The model under review builds one solid part; all positions refer to its coordinate system, in mm. Face numbers are marked on the shaded views. A direction names the side the tool comes from. Give positions to 0.01 mm unless a question says otherwise; leave off trailing zeros. Order: outer loops, then holes, each group sorted by start corner. A loop starts at its lowest first (then second) coordinate and runs counter-clockwise, first axis right, second up. Notation, with made-up numbers: M 64,17.25 L 76,17.25 A13 ccw 76,37.25 Z; hole C 23,18.5 d3. An arc over 180 degrees is marked long. One line per question, with ' | ' between items. Start each with the question number.
1. We need section C-C on x = 13. Write out the cut boundary in (y, z).
2. We need section A-A on z = -3. Write out the cut boundary in (x, y), then the cut area to 3 significant figures.
3. Wall thickness on L1, parallel to Z at x = 1, y = 18.5; L2, parallel to X at y = 13.5, z = -5; L3, parallel to Z at x = 10, y = 6 (3 decimals): over which ranges is each line inside the solid? List them lowest first.
4. For the marked faces 1 and 2, list the 3-axis set-ups (+Z, -Z, +X, -X, +Y, -Y) from which the entire face can be reached by the end or side of a thin tool; tool diameter is ignored.
5. The part is to be moulded in two halves that separate along Z. For the marked faces 3, 4 and 5, say which applies: +Z half, -Z half, draft (parallel to the pull), parting line (faces both ways), or undercut.
6. Insertion check: P1, Ø3, axis at x = -2.5, y = 14, coming from the -Z side; P2, Ø12, axis at x = -7.5, y = 7.5, coming from the +Z side; P3, Ø2, axis at y = 5.5, z = -11, coming from the +X side; P4, Ø9, axis at x = 5.56, z = -9.43, coming from the -Y side. Each pin has a flat end and moves straight along its axis. Give the tip position at first contact, or say it passes through.
```python
from build123d import *

# Parameters (mm, degrees)
SKETCH5_R               = 30
BOSS_EXTRUDE1_DEPTH     = 20
SKETCH6_R               = 5.75
CUT_EXTRUDE1_DEPTH      = 50
CUT_EXTRUDE_THIN1_DEPTH = 50
SKETCH11_R              = 1.5
CUT_EXTRUDE2_DEPTH      = 35.227641189


with BuildPart() as part:
    # Sketch5 → Boss-Extrude1 (new body)
    with BuildSketch(Plane(origin=(0, 0, 0), x_dir=(1, 0, 0), z_dir=(0, 1, 0))):
        with Locations(Location((0, 0, 0), (0, 0, 270))):
            Circle(SKETCH5_R)
    extrude(amount=BOSS_EXTRUDE1_DEPTH)

    # Sketch6 → Cut-Extrude1 (cut)
    with BuildSketch(Plane(origin=(0, 20, 0), x_dir=(1, 0, 0), z_dir=(0, 1, 0))):
        with Locations(Location((5.564652455, 9.430649132, 0), (0, 0, 270))):
            Circle(SKETCH6_R)
        with Locations(Location((5.325305202, -9.567843252, 0), (0, 0, 270))):
            Circle(SKETCH6_R)
        with Locations(Location((-11.00819821, 0.138683741, 0), (0, 0, 270))):
            Circle(SKETCH6_R)
    extrude(amount=-CUT_EXTRUDE1_DEPTH, mode=Mode.SUBTRACT)

    # Sketch9 → Cut-Extrude-Thin1 (cut)
    with BuildSketch(Plane(origin=(0, 20, 0), x_dir=(1, 0, 0), z_dir=(0, 1, 0))):
        with BuildLine():
            ThreePointArc((-3.76991423, 9.548248089), (5.682251411, 18.765215817), (14.899219139, 9.313050176))
            Line((14.899219139, 9.313050176), (14.659871887, -9.685442209))
            ThreePointArc((14.659871887, -9.685442209), (5.207706246, -18.902409937), (-4.009261482, -9.450244295))
            Line((-4.009261482, -9.450244295), (-14.008468, -9.324272058))
            ThreePointArc((-14.008468, -9.324272058), (5.081734008, -28.901616455), (24.659078405, -9.811414447))
            Line((24.659078405, -9.811414447), (24.898425657, 9.187077938))
            ThreePointArc((24.898425657, 9.187077938), (5.808223649, 28.764422335), (-13.769120748, 9.674220327))
            Line((-13.769120748, 9.674220327), (-3.76991423, 9.548248089))
        make_face()
        with BuildLine():
            ThreePointArc((10.124185438, -1.49260411), (13.400544345, -14.366723488), (0.526424967, -17.643082394))
            Line((0.526424967, -17.643082394), (-15.807078446, -7.936555401))
            ThreePointArc((-15.807078446, -7.936555401), (-19.083437352, 4.937563977), (-6.209317974, 8.213922883))
            Line((-6.209317974, 8.213922883), (-1.100619557, 16.810503626))
            ThreePointArc((-1.100619557, 16.810503626), (-27.680018096, 10.046262394), (-20.915776863, -16.533136145))
            Line((-20.915776863, -16.533136145), (-4.582273451, -26.239663138))
            ThreePointArc((-4.582273451, -26.239663138), (21.997125088, -19.475421905), (15.232883856, 7.103976633))
            Line((15.232883856, 7.103976633), (10.124185438, -1.49260411))
        make_face()
        with BuildLine():
            ThreePointArc((-6.438623457, -8.011462842), (-19.158344793, -4.430891012), (-15.577772963, 8.288830324))
            Line((-15.577772963, 8.288830324), (0.995077701, 17.580795716))
            ThreePointArc((0.995077701, 17.580795716), (13.714799038, 14.000223886), (10.134227208, 1.280502549))
            Line((10.134227208, 1.280502549), (15.024735309, -7.442050432))
            ThreePointArc((15.024735309, -7.442050432), (22.437352019, 18.890731987), (-3.8954304, 26.303348697))
            Line((-3.8954304, 26.303348697), (-20.468281064, 17.011383305))
            ThreePointArc((-20.468281064, 17.011383305), (-27.880897775, -9.321399113), (-1.548115356, -16.734015824))
            Line((-1.548115356, -16.734015824), (-6.438623457, -8.011462842))
        make_face()
    extrude(amount=-CUT_EXTRUDE_THIN1_DEPTH, mode=Mode.SUBTRACT)


with BuildPart() as cut_extrude_thin1_kept_piece:
    # of the separate pieces the step leaves, the one the design keeps (cut_extrude_thin1_pieces_kept)
    add(part.part.solids().sort_by_distance((-4.009261482, 0, 9.450244295))[0])

    # Sketch11 → Cut-Extrude2 (cut, through all)
    with BuildSketch(Plane(origin=(0, 20, 0), x_dir=(1, 0, 0), z_dir=(0, 1, 0))):
        with Locations(Location((0, 0, 0), (0, 0, 270))):
            Circle(SKETCH11_R)
    extrude(amount=-CUT_EXTRUDE2_DEPTH, mode=Mode.SUBTRACT)


solid = cut_extrude_thin1_kept_piece.part
```
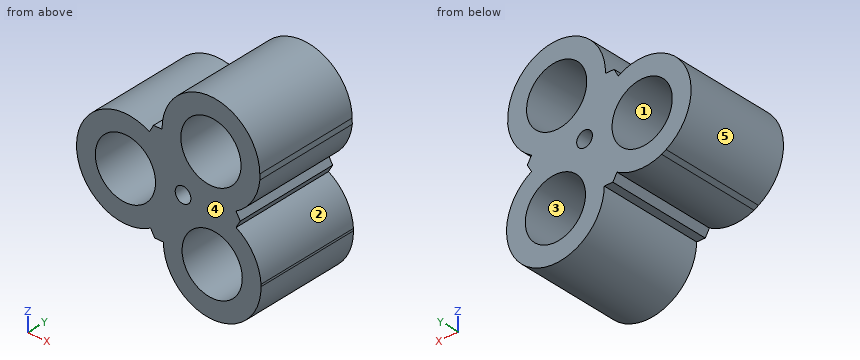
Entries:
1) outline: M 0,-15.08 L 20,-15.08 L 20,-3.77 L 0,-3.77 Z; M 0,4.15 L 20,4.15 L 20,14.88 L 0,14.88 Z
2) outline: M -19.9,0 L -16,0 L -16,20 L -19.9,20 Z; M -6.02,0 L 12.34,0 L 12.34,20 L -6.02,20 Z | area: 445 mm^2
3) L1: z = -17.57 to -12.93, -5.93 to -1.12, 1.12 to 5.78, 13.36 to 17.84 | L2: x = -18.99 to -14.08, -7.94 to 1.9, 9.23 to 13.79 | L3: z = -17.645 to -13.09, -5.771 to 6.22, 12.916 to 17.648
4) face 1: +Y, -Y | face 2: +X, +Y, -Y
5) face 3: undercut | face 4: draft | face 5: parting line
6) P1: stops at z = -16.07 | P2: stops at z = 15.94 | P3: stops at x = 14.88 | P4: passes through
